Read the model definition and answer for the solid it produces. Units are mm, in the model's axes. Face numbers are marked on the shaded views. A direction names the side the tool comes from. Give positions to 0.01 mm unless a question says otherwise; leave off trailing zeros. Put each result on its own line as item: value. Start each with the question number.
1. For the marked faces 5, 6, 7, 8 and 9, determine the directions among +Z, -Z, +X, -X, +Y, -Y from which every point of the face is accessible in a straight line to the end or side of a thin tool.
2. Consider L1, parallel to Z at x = -7.5, y = 18; L2, parallel to Y at x = 16, z = 4.5; L3, parallel to Y at x = 0, z = 3 (3 decimals). Determine where each line is inside the solid, lowest interval first. Write a range as from..to.
3. Given pin 1 Ø1 at (y, z) = (-18.5, 3) entering from +X; pin 2 Ø6 at (y, z) = (4.5, 6.5) entering from -X; pin 3 Ø10 at (x, y) = (-9, 15.5) entering from +Z (3 decimals); pin 4 Ø1.5 at (y, z) = (-12.5, 12.5) entering from +X, each flat-ended and moving along its own axis, determine where each tip first touches the part or whether it passes through.
4. For a pull along X with two mould halves and no side action, classify the marked faces 1, 2, 3 and 4 as released by +X, released by -X, zero draft, split by the parting line, or undercut.
5. A cutting plane is placed at D-D, the plane x = 12.5. Count the separate pieces of the cut face and the enclosed holes in it, plus the area to 3 significant figures.
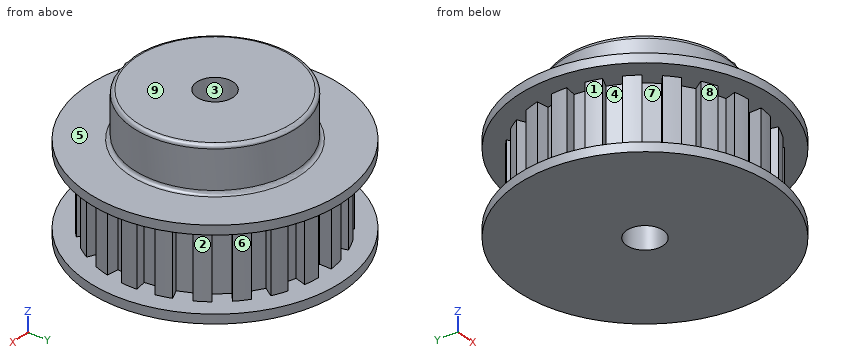
```python
from build123d import *

# Parameters (mm, degrees)
SKETCH1_R           = 3.175
BOSS_EXTRUDE3_DEPTH = 6.35
SKETCH2_R           = 22.225
SKETCH2_R_2         = 3.175
BOSS_EXTRUDE4_DEPTH = 1.5875
SKETCH3_R           = 14.2875
SKETCH3_R_2         = 3.175
BOSS_EXTRUDE5_DEPTH = 7.9375
FILLET1_R           = 0.635


with BuildPart() as part:
    # Sketch1 → Boss-Extrude3 (new body)
    with BuildSketch(Plane.XY):
        with BuildLine():
            Line((3.998939094, 18.625546599), (3.431060125, 16.691528444))
            Line((3.431060125, 16.691528444), (6.137730131, 15.896778422))
            Line((6.137730131, 15.896778422), (6.705609099, 17.830796578))
            ThreePointArc((6.705609099, 17.830796578), (7.913655998, 17.328489512), (9.084376828, 16.744449756))
            Line((9.084376828, 16.744449756), (7.994625068, 15.048762919))
            Line((7.994625068, 15.048762919), (10.367748965, 13.523648797))
            Line((10.367748965, 13.523648797), (11.457500725, 15.219335634))
            ThreePointArc((11.457500725, 15.219335634), (12.475096982, 14.397029391), (13.433852379, 13.506817177))
            Line((13.433852379, 13.506817177), (11.910513034, 12.186836121))
            Line((11.910513034, 12.186836121), (13.757834437, 10.054913573))
            Line((13.757834437, 10.054913573), (15.281173782, 11.37489463))
            ThreePointArc((15.281173782, 11.37489463), (16.0258798, 10.299207573), (16.694997104, 9.174942598))
            Line((16.694997104, 9.174942598), (14.861482068, 8.337604338))
            Line((14.861482068, 8.337604338), (16.033341984, 5.771589051))
            Line((16.033341984, 5.771589051), (17.86685702, 6.608927312))
            ThreePointArc((17.86685702, 6.608927312), (18.278341147, 5.367005208), (18.603612453, 4.099768736))
            Line((18.603612453, 4.099768736), (16.60846221, 3.812909438))
            Line((16.60846221, 3.812909438), (17.009923518, 1.020684709))
            Line((17.009923518, 1.020684709), (19.005073761, 1.307544008))
            ThreePointArc((19.005073761, 1.307544008), (19.05, 0), (19.005073761, -1.307544008))
            Line((19.005073761, -1.307544008), (17.009923518, -1.020684709))
            Line((17.009923518, -1.020684709), (16.60846221, -3.812909438))
            Line((16.60846221, -3.812909438), (18.603612453, -4.099768736))
            ThreePointArc((18.603612453, -4.099768736), (18.278341147, -5.367005208), (17.86685702, -6.608927312))
            Line((17.86685702, -6.608927312), (16.033341984, -5.771589051))
            Line((16.033341984, -5.771589051), (14.861482068, -8.337604338))
            Line((14.861482068, -8.337604338), (16.694997104, -9.174942598))
            ThreePointArc((16.694997104, -9.174942598), (16.0258798, -10.299207573), (15.281173782, -11.37489463))
            Line((15.281173782, -11.37489463), (13.757834437, -10.054913573))
            Line((13.757834437, -10.054913573), (11.910513034, -12.186836121))
            Line((11.910513034, -12.186836121), (13.433852379, -13.506817177))
            ThreePointArc((13.433852379, -13.506817177), (12.475096982, -14.397029391), (11.457500725, -15.219335634))
            Line((11.457500725, -15.219335634), (10.367748965, -13.523648797))
            Line((10.367748965, -13.523648797), (7.994625068, -15.048762919))
            Line((7.994625068, -15.048762919), (9.084376828, -16.744449756))
            ThreePointArc((9.084376828, -16.744449756), (7.913655998, -17.328489512), (6.705609099, -17.830796578))
            Line((6.705609099, -17.830796578), (6.137730131, -15.896778422))
            Line((6.137730131, -15.896778422), (3.431060125, -16.691528444))
            Line((3.431060125, -16.691528444), (3.998939094, -18.625546599))
            ThreePointArc((3.998939094, -18.625546599), (2.711097669, -18.856098468), (1.410468904, -18.997712427))
            Line((1.410468904, -18.997712427), (1.410468904, -16.982045602))
            Line((1.410468904, -16.982045602), (-1.410468904, -16.982045602))
            Line((-1.410468904, -16.982045602), (-1.410468904, -18.997712427))
            ThreePointArc((-1.410468904, -18.997712427), (-2.711097669, -18.856098468), (-3.998939094, -18.625546599))
            Line((-3.998939094, -18.625546599), (-3.431060125, -16.691528444))
            Line((-3.431060125, -16.691528444), (-6.137730131, -15.896778422))
            Line((-6.137730131, -15.896778422), (-6.705609099, -17.830796578))
            ThreePointArc((-6.705609099, -17.830796578), (-7.913655998, -17.328489512), (-9.084376828, -16.744449756))
            Line((-9.084376828, -16.744449756), (-7.994625068, -15.048762919))
            Line((-7.994625068, -15.048762919), (-10.367748965, -13.523648797))
            Line((-10.367748965, -13.523648797), (-11.457500725, -15.219335634))
            ThreePointArc((-11.457500725, -15.219335634), (-12.475096982, -14.397029391), (-13.433852379, -13.506817177))
            Line((-13.433852379, -13.506817177), (-11.910513034, -12.186836121))
            Line((-11.910513034, -12.186836121), (-13.757834437, -10.054913573))
            Line((-13.757834437, -10.054913573), (-15.281173782, -11.37489463))
            ThreePointArc((-15.281173782, -11.37489463), (-16.0258798, -10.299207573), (-16.694997104, -9.174942598))
            Line((-16.694997104, -9.174942598), (-14.861482068, -8.337604338))
            Line((-14.861482068, -8.337604338), (-16.033341984, -5.771589051))
            Line((-16.033341984, -5.771589051), (-17.86685702, -6.608927312))
            ThreePointArc((-17.86685702, -6.608927312), (-18.278341147, -5.367005208), (-18.603612453, -4.099768736))
            Line((-18.603612453, -4.099768736), (-16.60846221, -3.812909438))
            Line((-16.60846221, -3.812909438), (-17.009923518, -1.020684709))
            Line((-17.009923518, -1.020684709), (-19.005073761, -1.307544008))
            ThreePointArc((-19.005073761, -1.307544008), (-19.05, 0), (-19.005073761, 1.307544008))
            Line((-19.005073761, 1.307544008), (-17.009923518, 1.020684709))
            Line((-17.009923518, 1.020684709), (-16.60846221, 3.812909438))
            Line((-16.60846221, 3.812909438), (-18.603612453, 4.099768736))
            ThreePointArc((-18.603612453, 4.099768736), (-18.278341147, 5.367005208), (-17.86685702, 6.608927312))
            Line((-17.86685702, 6.608927312), (-16.033341984, 5.771589051))
            Line((-16.033341984, 5.771589051), (-14.861482068, 8.337604338))
            Line((-14.861482068, 8.337604338), (-16.694997104, 9.174942598))
            ThreePointArc((-16.694997104, 9.174942598), (-16.0258798, 10.299207573), (-15.281173782, 11.37489463))
            Line((-15.281173782, 11.37489463), (-13.757834437, 10.054913573))
            Line((-13.757834437, 10.054913573), (-11.910513034, 12.186836121))
            Line((-11.910513034, 12.186836121), (-13.433852379, 13.506817177))
            ThreePointArc((-13.433852379, 13.506817177), (-12.475096982, 14.397029391), (-11.457500725, 15.219335634))
            Line((-11.457500725, 15.219335634), (-10.367748965, 13.523648797))
            Line((-10.367748965, 13.523648797), (-7.994625068, 15.048762919))
            Line((-7.994625068, 15.048762919), (-9.084376828, 16.744449756))
            ThreePointArc((-9.084376828, 16.744449756), (-7.913655998, 17.328489512), (-6.705609099, 17.830796578))
            Line((-6.705609099, 17.830796578), (-6.137730131, 15.896778422))
            Line((-6.137730131, 15.896778422), (-3.431060125, 16.691528444))
            Line((-3.431060125, 16.691528444), (-3.998939094, 18.625546599))
            ThreePointArc((-3.998939094, 18.625546599), (-2.711097669, 18.856098468), (-1.410468904, 18.997712427))
            Line((-1.410468904, 18.997712427), (-1.410468904, 16.982045602))
            Line((-1.410468904, 16.982045602), (1.410468904, 16.982045602))
            Line((1.410468904, 16.982045602), (1.410468904, 18.997712427))
            ThreePointArc((1.410468904, 18.997712427), (2.711097669, 18.856098468), (3.998939094, 18.625546599))
        make_face()
        Circle(SKETCH1_R, mode=Mode.SUBTRACT)
    boss_extrude3 = extrude(amount=BOSS_EXTRUDE3_DEPTH)

    # Sketch2 → Boss-Extrude4 (add)
    with BuildSketch(Plane.XY.offset(6.35)):
        Circle(SKETCH2_R)
        Circle(SKETCH2_R_2, mode=Mode.SUBTRACT)
    boss_extrude4 = extrude(amount=BOSS_EXTRUDE4_DEPTH)

    # Sketch3 → Boss-Extrude5 (add)
    with BuildSketch(Plane.XY.offset(7.9375)):
        Circle(SKETCH3_R)
        Circle(SKETCH3_R_2, mode=Mode.SUBTRACT)
    extrude(amount=BOSS_EXTRUDE5_DEPTH)

    # Fillet1
    fillet1_edges = [part.edges().sort_by_distance(p)[0] for p in [
        (-14.2875, 0, 7.9375),
        (-14.2875, 0, 15.875),
    ]]
    fillet(fillet1_edges, radius=FILLET1_R)

    # Mirror1: Boss-Extrude3, Boss-Extrude4 across plane
    add(boss_extrude3.mirror(Plane.XY))
    add(boss_extrude4.mirror(Plane.XY))


solid = part.part
```
Return value:
1. face 5: +Z
1. face 6: +X, +Y
1. face 7: none
1. face 8: -X, -Y
1. face 9: +Z, +X, -X, +Y, -Y
2. L1: z = -7.94..-6.35, 6.35..7.94
2. L2: y = -10.34..-8.86, -5.84..5.84, 8.86..10.34
2. L3: y = -16.982..-3.175, 3.175..16.982
3. pin 1: stops at x = 4
3. pin 2: stops at x = -22.17
3. pin 3: stops at z = 15.875
3. pin 4: stops at x = 8.13
4. face 1: released by -X
4. face 2: released by +X
4. face 3: undercut
4. face 4: undercut
5. separate pieces: 1
5. enclosed holes: 2
5. area: 561 mm2
